Solid Edge part; units mm, degrees
sketch "Sketch1" plane through (0, 0, 0) normal (0, 0, 1) x (1, 0, 0)
  circle A0 centre (0, 0) radius 4.25
extrude "Protrusion1" add sketch "Sketch1" along normal blind 5
sketch "Sketch2" plane through (0, 0, 0) normal (0, 0, -1) x (1, 0, 0)
  circle A0 centre (0, 0) radius 2.5
extrude "Protrusion2" add sketch "Sketch2" along normal blind 75
sketch "Sketch3" plane through (0, 0, -75) normal (0, 0, -1) x (1, 0, 0)
  circle A0 centre (0, 0) radius 2.4997
extrude "Cutout1" cut sketch "Sketch3" against normal blind 22 flip side to cut
chamfer "Chamfer_1" distance 0.375 angle 45 1 edges at (-2.4997, 0, -75)
sketch "Sketch4" plane through (0, 0, 5) normal (0, 0, 1) x (1, 0, 0)
  line L0 (-1.1547, 2) -> (1.1547, 2)
  line L1 (2.3094, 0) -> (1.1547, 2)
  line L2 (1.1547, -2) -> (2.3094, 0)
  line L3 (-1.1547, -2) -> (1.1547, -2)
  line L4 (-2.3094, 0) -> (-1.1547, -2)
  line L5 (-1.1547, 2) -> (-2.3094, 0)
extrude "Cutout2" cut sketch "Sketch4" against normal blind 2.5
properties part number "185705" material "Stainless Steel, 304"
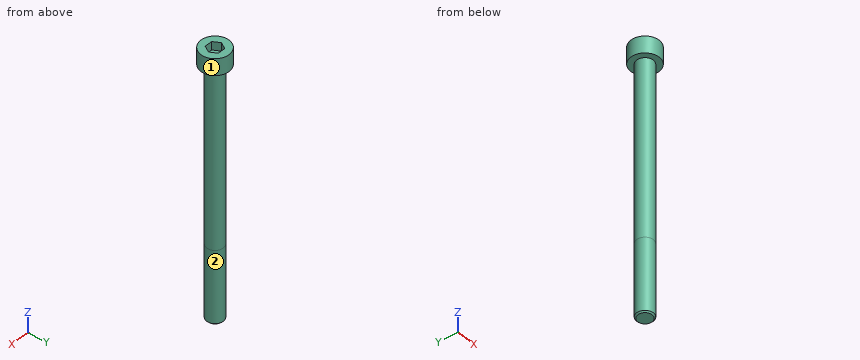
Input: part model. Units: mm. Frame: model coordinates. Face numbers are marked on the shaded views. A direction names the side the tool comes from. Coordinates: 2 decimals unless noted, no trailing zeros. Write each loop counter-clockwise with the first axis right and the second up, starting at its lowest first coordinate (ties: lowest second). Pieces come first, ordered by that corner, then holes. Notation, with made-up numbers: (34.5, -32.75) - (71.5, -32.75) arc R29 cw to (71.5, -4.75) - close; hole circle Ø7 at (-11.75, 15). An arc over 180 degrees is marked (long way). Put each result on its own line as item: value. Start each with the question number.
1) Ray query, L1, parallel to Y at x = 0, z = -19; L2, parallel to Z at x = -2.5, y = 3. Return the intervals inside material, ascending.
2) Contact query for flat-ended pins moving along their axis: pin 1 (1 mm diameter, centred on y = -2, z = -20.5, fed in from -X); pin 2 (4 mm diameter, centred on x = -2.5, z = -16, fed in from +Y); pin 3 (1 mm diameter, centred on x = 1, z = -40.5, fed in from -Y). Output: stop coordinate, or through.
3) Reachability of the marked faces 1 and 2 from +Z, -Z, +X, -X, +Y, -Y: full face, straight path, thin tool, end or side. Return the list, or none.
4) Cut plane B-B (z = -15). Return the cut outline in (x, y).
Resolved:
1. L1: y = -2.5 to 2.5
1. L2: z = 0 to 5
2. pin 1: stops at x = -2
2. pin 2: stops at y = 2.45
2. pin 3: stops at y = -2.45
3. face 1: +Z, -Z
3. face 2: -Z
4. outline: circle Ø5 at (0, 0)
